Autodesk Inventor part; units mm, degrees
ref_plane "YZ Plane" through (0, 0, 0) normal (1, 0, 0) x (0, 1, 0)
ref_plane "XZ Plane" through (0, 0, 0) normal (0, 1, 0) x (-1, 0, 0)
ref_plane "XY Plane" through (0, 0, 0) normal (0, 0, 1) x (1, 0, 0)
sketch "Sketch1" plane through (0, 0, 0) normal (0, 1, 0) x (-1, 0, 0)
  line L0 (420, 0) -> (-420, 0)
  line L1 (0, 50) -> (-10, 50)
  line L2 (0, -50) -> (-10, -50)
  line L3 (-10, -50) -> (-300, 0)
  line L4 (-300, 0) -> (-10, 50)
  line L5 (0, 50) -> (0, -50)
  line L6 (0, 50) -> (10, 50)
  line L7 (0, -50) -> (10, -50)
  line L8 (10, -50) -> (300, 0)
  line L9 (300, 0) -> (10, 50)
  line L10 (-300, 0) -> (300, 0)
  line L11 (0, -70) -> (0, 70)
  line L12 (-300, 0) -> (-300, 0)
  line L13 (300, 0) -> (300, 0)
  line L14 (0, 42) -> (9.3154, 42)
  line L15 (9.3154, 42) -> (252.9154, 0)
  line L16 (252.9154, 0) -> (9.3154, -42)
  line L17 (9.3154, -42) -> (0, -42)
  line L18 (0, 42) -> (-9.3154, 42)
  line L19 (-9.3154, 42) -> (-252.9154, 0)
  line L20 (-252.9154, 0) -> (-9.3154, -42)
  line L21 (-9.3154, -42) -> (0, -42)
  line L22 (9.3154, 42) -> (9.3154, -42)
  line L23 (-9.3154, 42) -> (-9.3154, -42)
  point P0 (0, 0)
  point P1 (300, 0)
  point P2 (-300, 0)
  dimension "d36" = 600
  dimension "d38" = 10
  dimension "d39" = 100
  dimension "d44" = 8
  dimension "d45" = 8
  dimension "d47" = 600
  dimension "d49" = 300
  dimension "d51" = 0
  dimension "d52" = 300
  dimension "d53" = 300
  dimension "d54" = 0
  dimension "d55" = 0
  dimension "d56" = 0
  dimension "d57" = 0
  dimension "d60" = 0
extrude "Main_block" add sketch "Sketch1" along normal blind 6.35 contours L8 L7 L5 L17 L16 L0 | L0 L15 L14 L5 L6 L9 | L22 L17 L5 L0 | L0 L5 L14 L22 | L2 L3 L0 L20 L21 L5 | L5 L18 L19 L0 L4 L1 | L5 L21 L23 L0 | L0 L23 L18 L5
fillet "Fillet7" radius 4 6 edges at (-9.3154, 3.175, -42) (9.3154, 3.175, -42) (9.3154, 3.175, 42) (-9.3154, 3.175, 42) (252.9154, 3.175, 0) (-252.9154, 3.175, 0)
sketch "Sketch4" plane through (0, 6.35, 0) normal (0, 1, 0) x (1, 0, 0)
  line L0 (-300, 0) -> (-10, -50)
  line L1 (-10, 50) -> (-300, 0)
  line L2 (-275, 4.3103) -> (-275, -4.3103)
  line L3 (-275, -4.3103) -> (-300, 0)
  line L4 (-300, 0) -> (-275, 4.3103)
  line L5 (0, 70) -> (0, -70)
  line L6 (275, 4.3103) -> (275, -4.3103)
  line L7 (275, -4.3103) -> (300, 0)
  line L8 (300, 0) -> (275, 4.3103)
  point P0 (0, 0)
extrude "Extrusion4" cut sketch "Sketch4" against normal blind 10
properties part number "Main Support"
The model under review builds one solid part; all positions refer to its coordinate system, in mm. A direction names the side the tool comes from. Give positions to 0.01 mm unless a question says otherwise; leave off trailing zeros. Write each loop counter-clockwise with the first axis right and the second up, starting at its lowest first coordinate (ties: lowest second). Pieces come first, ordered by that corner, then holes. Notation, with made-up numbers: (86, 80) -> (102, 80) arc R21 cw to (102, 113) -> close; hole circle Ø10 at (68.5, 87.25). An arc over 180 degrees is marked (long way). Answer in a Markdown table with one row per item.
1) Tool access review of faces 1 (the flat face through (123.536, 3.131, -22.307)), 2 (the flat face through (-144.355, 3.131, 26.835)): name each direction out of +Z, -Z, +X, -X, +Y, -Y from which nothing blocks a thin tool from reaching the whole face with its end or side.
Worked answers:
| item | result |
|---|---|
| face 1 | +Y, -Y |
| face 2 | +Z, -X, +Y, -Y |
2) Clearance check with a flat-ended pin moving along its axis: P1, Ø2, axis at x = -80, y = 1.5, coming from the +Z side. State where the tip first meets the part, or that it passes through.
Worked answers:
| item | result |
|---|---|
| P1 | z = 38.1 |
3) Add section C-C on y = 4. State the section outline as (x, z) points, plus the area to 3 significant figures.
Worked answers:
| item | result |
|---|---|
| outline | (-275, -4.31) -> (-10, -50) -> (10, -50) -> (275, -4.31) -> (275, 4.31) -> (10, 50) -> (-10, 50) -> (-275, 4.31) -> close; hole (-230.05, -3.94) -> (-14, -41.19) arc R4 ccw to (-9.32, -37.25) -> (-9.32, 37.25) arc R4 ccw to (-14, 41.19) -> (-230.05, 3.94) arc R4 ccw to start; hole (9.32, -37.25) arc R4 ccw to (14, -41.19) -> (230.05, -3.94) arc R4 ccw to (230.05, 3.94) -> (14, 41.19) arc R4 ccw to (9.32, 37.25) -> close |
| area | 10,500 mm² |
4) Mouldability with a two-part tool opening along Z and no side actions: class faces 3 (the flat face through (140.645, 3.131, -27.475)), 4 (the flat face through (144.355, 3.131, 26.835)), 5 (the flat face through (-120.51, 3.13, 22.83)), 6 (the flat face through (1, 6.35, 0)) as +Z half, -Z half, draft (parallel to the pull), parting line (faces both ways), or undercut.
Worked answers:
| item | result |
|---|---|
| face 3 | -Z half |
| face 4 | +Z half |
| face 5 | undercut |
| face 6 | draft |
5) Add section A-A on x = -139. State the section outline as (y, z) points, plus the area to 3 significant figures.
Worked answers:
| item | result |
|---|---|
| outline | (0, -27.76) -> (6.35, -27.76) -> (6.35, -19.64) -> (0, -19.64) -> close; (0, 19.64) -> (6.35, 19.64) -> (6.35, 27.76) -> (0, 27.76) -> close |
| area | 103 mm² |
6) For L1, parallel to X at y = 0.5, z = 1; L2, parallel to Z at x = 221, y = 2.5; L3, parallel to Z at x = 45.5, y = 1.5, list the stretches that pass through material, from the lowest coordinate up. Write a range as [from, to].
Worked answers:
| item | result |
|---|---|
| L1 | [-275, -233.25], [-9.32, 9.32], [233.25, 275] |
| L2 | [-13.62, -5.5], [5.5, 13.62] |
| L3 | [-43.88, -35.76], [35.76, 43.88] |
7) Add section B-B on z = 32.5. State the section outline as (x, y) points.
Worked answers:
| item | result |
|---|---|
| outline | (-111.5, 0) -> (-64.42, 0) -> (-64.42, 6.35) -> (-111.5, 6.35) -> close; (-9.32, 0) -> (9.32, 0) -> (9.32, 6.35) -> (-9.32, 6.35) -> close; (64.42, 0) -> (111.5, 0) -> (111.5, 6.35) -> (64.42, 6.35) -> close |
